from build123d import *

# Parameters (mm, degrees)
BOSS_EXTRUDE1_DEPTH = 37.5
FILLET1_R           = 5
CHAMFER1_SIZE       = 2.5


with BuildPart() as part:
    # Sketch1 → Boss-Extrude1 (new body, symmetric)
    with BuildSketch(Plane(origin=(0, 0, 0), x_dir=(1, 0, 0), z_dir=(0, 1, 0))):
        with BuildLine():
            Line((-97.927346189, 41.968862652), (77.072653811, -33.031137348))
            Line((77.072653811, -33.031137348), (47.38494666, -33.031137348))
            ThreePointArc((47.38494666, -33.031137348), (43.302463755, -32.159846639), (39.931386735, -29.697804014))
            ThreePointArc((39.931386735, -29.697804014), (36.204606772, -28.031137348), (32.47782681, -29.697804014))
            ThreePointArc((32.47782681, -29.697804014), (29.106749789, -32.159846639), (25.024266885, -33.031137348))
            Line((25.024266885, -33.031137348), (0.752993699, -33.031137348))
            ThreePointArc((0.752993699, -33.031137348), (-3.329489206, -32.159846639), (-6.700566226, -29.697804014))
            ThreePointArc((-6.700566226, -29.697804014), (-10.427346189, -28.031137348), (-14.154126151, -29.697804014))
            ThreePointArc((-14.154126151, -29.697804014), (-17.525203172, -32.159846639), (-21.607686076, -33.031137348))
            Line((-21.607686076, -33.031137348), (-42.33546369, -33.031137348))
            ThreePointArc((-42.33546369, -33.031137348), (-46.417946594, -32.159846639), (-49.789023615, -29.697804014))
            ThreePointArc((-49.789023615, -29.697804014), (-53.515803577, -28.031137348), (-57.24258354, -29.697804014))
            ThreePointArc((-57.24258354, -29.697804014), (-60.61366056, -32.159846639), (-64.696143465, -33.031137348))
            Line((-64.696143465, -33.031137348), (-97.927346189, -33.031137348))
            Line((-97.927346189, -33.031137348), (-97.927346189, 41.968862652))
        make_face()
    extrude(amount=BOSS_EXTRUDE1_DEPTH, both=True)

    # Fillet1
    fillet1_edges = [part.edges().sort_by_distance(p)[0] for p in [
        (-97.927346189, 0, 33.031137348),
        (-97.927346189, 0, -41.968862652),
        (77.072653811, 0, 33.031137348),
    ]]
    fillet(fillet1_edges, radius=FILLET1_R)

    # Chamfer1
    chamfer1_edges = [part.edges().sort_by_distance(p)[0] for p in [
        (43.302463755, -37.5, 32.159846639),
        (36.204606772, -37.5, 28.031137348),
        (29.106749789, -37.5, 32.159846639),
        (12.888630292, -37.5, 33.031137348),
        (-3.329489206, -37.5, 32.159846639),
        (-10.427346189, -37.5, 28.031137348),
        (-17.525203172, -37.5, 32.159846639),
        (-31.971574883, -37.5, 33.031137348),
        (-46.417946594, -37.5, 32.159846639),
        (-53.515803577, -37.5, 28.031137348),
        (-60.61366056, -37.5, 32.159846639),
        (50.048989314, -37.5, 33.031137348),
        (-60.61366056, 37.5, 32.159846639),
        (-53.515803577, 37.5, 28.031137348),
        (-46.417946594, 37.5, 32.159846639),
        (-31.971574883, 37.5, 33.031137348),
        (-17.525203172, 37.5, 32.159846639),
        (-10.427346189, 37.5, 28.031137348),
        (-18.137560617, -37.5, -7.773240265),
        (-18.137560617, 37.5, -7.773240265),
        (-3.329489206, 37.5, 32.159846639),
        (-78.811744827, -37.5, 33.031137348),
        (-97.927346189, -37.5, -3.177515114),
        (-95.679801232, -37.5, -38.560373038),
        (-96.462880095, -37.5, 31.566671254),
        (57.610920582, -37.5, 29.036466709),
        (-97.927346189, 37.5, -3.177515114),
        (12.888630292, 37.5, 33.031137348),
        (-78.811744827, 37.5, 33.031137348),
        (-95.679801232, 37.5, -38.560373038),
        (-96.462880095, 37.5, 31.566671254),
        (50.048989314, 37.5, 33.031137348),
        (57.610920582, 37.5, 29.036466709),
        (29.106749789, 37.5, 32.159846639),
        (36.204606772, 37.5, 28.031137348),
        (43.302463755, 37.5, 32.159846639),
    ]]
    chamfer(chamfer1_edges, length=CHAMFER1_SIZE)


solid = part.part
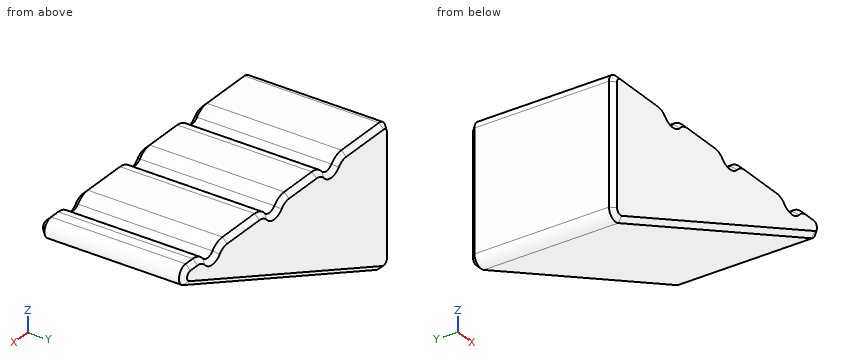
The listing builds one solid part. Answer for the finished solid, in the listing's coordinates (mm). Round coordinates to 2 decimals unless told otherwise and drop trailing zeros. Write each loop counter-clockwise with the first axis right and the second up, starting at its lowest first coordinate (ties: lowest second). Pieces come first, ordered by that corner, then holes. Notation, with made-up numbers: M 18,-5 L 71,-5 A30 ccw 71,17 Z; hole C 26.25,36 d4. An arc over 180 degrees is marked long. Write each question's results on one line, items separated by ' | '. Start each with the question number.
(1) Each of these flat-tipped pins is pushed along its axis until it touches: P1, Ø4, axis at x = 40, y = 25, coming from the +Z side; P2, Ø1, axis at y = 14, z = -10.5, coming from the +X side; P3, Ø2, axis at y = 13, z = -17, coming from the +X side. Where does it stop, or does it pass through?
(2) The part is cut by section C-C, the plane x = 20. Write down the section's boundary in (y, z), and give its area (3 significant figures).
(3) Find the intervals of material crossed by line 1 (Z direction, x = -79, y = 30.5); line 2 (Z direction, x = -45, y = -8.5); line 3 (X direction, y = -20, z = -25), in increasing order.
(4) The part is cut by section A-A, the plane y = 4.5. Write down the section's boundary in (x, z), and give its area (3 significant figures).
(5) The part is cut by section B-B, the plane z = -17. Write down the section's boundary in (x, y).
Worked answers:
1) P1: stops at z = 31.46 | P2: stops at x = -23.33 | P3: stops at x = -37.33
2) outline: M -37.5,11.29 L -35,8.57 L 35,8.57 L 37.5,11.29 L 37.5,30.53 L 35,33.03 L -35,33.03 L -37.5,30.53 Z | area: 1,820 mm²
3) line 1: z = -33.86 to 33.03 | line 2: z = -19.29 to 32.67 | line 3: x = -97.93 to -58.33
4) outline: M -97.93,-34.39 A5 ccw -90.96,-38.98 L 54.68,23.44 A5 ccw 52.71,33.03 L 47.38,33.03 A10 ccw 39.93,29.7 A5 cw 32.48,29.7 A10 ccw 25.02,33.03 L 0.75,33.03 A10 ccw -6.7,29.7 A5 cw -14.15,29.7 A10 ccw -21.61,33.03 L -42.34,33.03 A10 ccw -49.79,29.7 A5 cw -57.24,29.7 A10 ccw -64.7,33.03 L -92.93,33.03 A5 ccw -97.93,28.03 Z | area: 6,310 mm²
5) outline: M -97.93,-35 L -95.43,-37.5 L -46.01,-37.5 L -39.67,-35 L -39.67,35 L -46.01,37.5 L -95.43,37.5 L -97.93,35 Z
